Build history of the part. All positions in model axes, mm. Face numbers are marked on the shaded views. A direction names the side the tool comes from. Round coordinates to 2 decimals unless told otherwise and drop trailing zeros. Write each loop counter-clockwise with the first axis right and the second up, starting at its lowest first coordinate (ties: lowest second). Pieces come first, ordered by that corner, then holes.
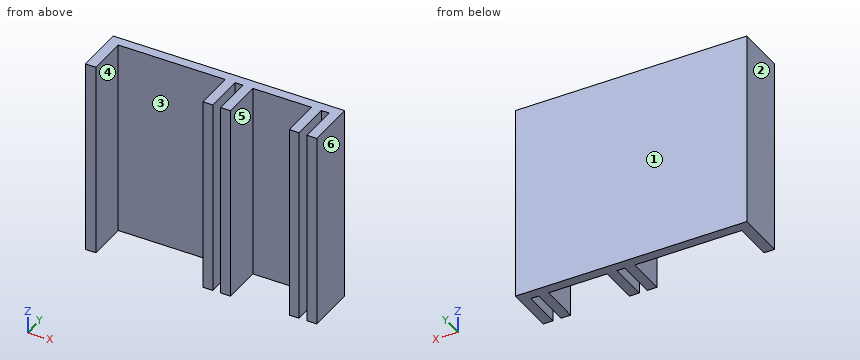
Autodesk Fusion 360 part; units mm, degrees
sketch "Sketch6" plane through (0, 0, 0) normal (0, 0, 1) x (1, 0, 0)
  line L0 (59, -2.5) -> (-59, -2.5)
  line L1 (-59, -2.5) -> (-59, 2.5)
  line L2 (-59, 2.5) -> (59, 2.5)
  line L3 (59, 2.5) -> (59, -2.5)
  line L4 (59, -2.5) -> (-59, 2.5) construction
  line L5 (-59, -2.5) -> (59, 2.5) construction
  dimension "d8" = 118
  dimension "d9" = 5
sketch "Sketch7" plane through (0, 0, 0) normal (0, 0, 1) x (1, 0, 0)
  line L0 (-464, -2.5) -> (-459, -2.5)
  line L1 (-459, -2.5) -> (-459, -22.5)
  line L2 (-459, -22.5) -> (-464, -22.5)
  line L3 (-464, -22.5) -> (-464, -2.5)
  line L4 (-459, -22.5) -> (-464, -22.5)
  line L5 (-464, -22.5) -> (-464, -2.5)
  line L6 (-459, -2.5) -> (-459, -22.5)
  line L7 (-464, -2.5) -> (-459, -2.5)
  dimension "d10" = 5
  dimension "d11" = 20
  dimension "d12" = 5
  dimension "d13" = 20
sketch "Sketch8" plane through (0, 0, 0) normal (0, 0, 1) x (1, 0, 0)
  line L0 (136, -2.5) -> (141, -2.5)
  line L1 (141, -2.5) -> (141, -22.5)
  line L2 (141, -22.5) -> (136, -22.5)
  line L3 (136, -22.5) -> (136, -2.5)
  dimension "d14" = 5
  dimension "d15" = 20
sketch "Sketch9" plane through (0, 0, 0) normal (0, 0, 1) x (1, 0, 0)
  line L0 (459, -2.5) -> (464, -2.5)
  line L1 (464, -2.5) -> (464, -22.5)
  line L2 (464, -22.5) -> (459, -22.5)
  line L3 (459, -22.5) -> (459, -2.5)
  dimension "d16" = 5
  dimension "d17" = 20
sketch "Sketch10" plane through (0, 0, 0) normal (0, 0, 1) x (1, 0, 0)
  line L0 (450, -2.5) -> (455, -2.5)
  line L1 (455, -2.5) -> (455, -22.5)
  line L2 (455, -22.5) -> (450, -22.5)
  line L3 (450, -22.5) -> (450, -2.5)
  dimension "d20" = 5
  dimension "d21" = 20
sketch "Sketch11" plane through (0, 0, 0) normal (0, 0, 1) x (1, 0, 0)
  line L0 (145, -2.5) -> (150, -2.5)
  line L1 (150, -2.5) -> (150, -22.5)
  line L2 (150, -22.5) -> (145, -22.5)
  line L3 (145, -22.5) -> (145, -2.5)
  dimension "d22" = 5
  dimension "d23" = 20
extrude "Extrude1" add sketch "Sketch6" along normal blind 100 makes body 1
extrude "Extrude2" add sketch "Sketch7" along normal blind 100 bodies 1 makes body 2
extrude "Extrude3" add sketch "Sketch8" along normal blind 100 bodies 2 makes body 3
extrude "Extrude4" add sketch "Sketch11" along normal blind 100 bodies 3 makes body 4
extrude "Extrude5" add sketch "Sketch10" along normal blind 100 bodies 4 makes body 5
extrude "Extrude6" add sketch "Sketch9" along normal blind 100 bodies 5 makes body 6
move_body "Move1" bodies 2 to x (1, 0, 0) y (0, 1, 0) z (0, 0, 1) at (418, 0, 0)
move_face "MoveFace1" by (-0.4, 0, 0) 1 faces at (-46, -15.8333, 33.3333) on bodies 2
move_body "Move2" bodies 5 6 to x (1, 0, 0) y (0, 1, 0) z (0, 0, 1) at (-417.6, 0, 0)
move_body "Move3" bodies 4 3 to x (1, 0, 0) y (0, 1, 0) z (0, 0, 1) at (-140, 0, 0)
move_body "Move4" bodies 3 4 to x (1, 0, 0) y (0, 1, 0) z (0, 0, 1) at (5, 0, 0)
move_body "Move5" bodies 4 3 to x (1, 0, 0) y (0, 1, 0) z (0, 0, 1) at (7, 0, 0)
move_body "Move6" bodies 4 3 to x (1, 0, 0) y (0, 1, 0) z (0, 0, 1) at (4, 0, 0)
move_body "Move7" bodies 2 to x (1, 0, 0) y (0, 1, 0) z (0, 0, 1) at (-12.6, 0, 0)
move_body "Move8" bodies 6 5 to x (1, 0, 0) y (0, 1, 0) z (0, 0, 1) at (12.6, 0, 0)
move_body "Move9" bodies 4 3 to x (1, 0, 0) y (0, 1, 0) z (0, 0, 1) at (-11, 0, 0)
combine "Combine1" operation add target body 1 tool bodies 2 3 4 6 5
1) Pin check, flat tips, straight feed: pin 1 Ø9 at (x, z) = (26, 38.5) entering from -Y; pin 2 Ø10 at (x, y) = (-9.5, -8) entering from -Z. Stop position of each tip, or through.
Results:
pin 1: stops at y = -2.5
pin 2: passes through
2) Wall check: L1, parallel to X at y = -18.25, z = 64; L2, parallel to Y at x = -18, z = 47. Give the ranges that are in metal, low to high.
Results:
L1: x = -59 to -53.6, 1 to 6, 10 to 15, 45 to 50, 54 to 59
L2: y = -2.5 to 2.5
3) Slice it at B-B (z = 91). Write the cut outline in (x, y), plus the area to 3 significant figures.
Results:
outline: (-59, -22.5) - (-53.6, -22.5) - (-53.6, -2.5) - (1, -2.5) - (1, -22.5) - (6, -22.5) - (6, -2.5) - (10, -2.5) - (10, -22.5) - (15, -22.5) - (15, -2.5) - (45, -2.5) - (45, -22.5) - (50, -22.5) - (50, -2.5) - (54, -2.5) - (54, -22.5) - (59, -22.5) - (59, 2.5) - (-59, 2.5) - close
area: 1,100 mm2
4) Which spindle directions (+Z, -Z, +X, -X, +Y, -Y) get a long thin tool onto all of the face, cutting with end or side? Do the marked faces 5 and 6. Say none if no direction does.
Results:
face 5: +Z, -Z, -Y
face 6: +Z, -Z, +X, +Y, -Y
5) Slice it at A-A (y = -11). Write the cut outline in (x, z), plus the area to 3 significant figures.
Results:
outline: (-59, 0) - (-53.6, 0) - (-53.6, 100) - (-59, 100) - close; (1, 0) - (6, 0) - (6, 100) - (1, 100) - close; (10, 0) - (15, 0) - (15, 100) - (10, 100) - close; (45, 0) - (50, 0) - (50, 100) - (45, 100) - close; (54, 0) - (59, 0) - (59, 100) - (54, 100) - close
area: 2,540 mm2
6) Slice it at C-C (x = -29). Write the cut outline in (y, z), plus the area to 3 significant figures.
Results:
outline: (-2.5, 0) - (2.5, 0) - (2.5, 100) - (-2.5, 100) - close
area: 500 mm2
7) Mould opens along X. For the marked faces 1, 2, 3 and 4 say: released by +X, released by -X, zero draft, split by the parting line, or undercut.
Results:
face 1: zero draft
face 2: released by -X
face 3: undercut
face 4: undercut
